Geometry check sheet. Reference: the model listing, model coordinates, mm. Give positions to 0.01 mm unless a question says otherwise; leave off trailing zeros. Write item = value, one per line. Start each with the question number.
1. Thickness scan on line 1 along X through (y, z) = (0.8, -6); line 2 along X through (y, z) = (0.6, -3); line 3 along Z through (x, y) = (-1.5, 1.25). Record the ranges inside material, lowest first.
2. Mould release check, pull along Z, two halves, no side actions. Record for faces 1 (the flat face through (4, 0, 13)), 2 (the conical face through (5.31, 2.94, -12.81)), 3 (the cylindrical face through (-13.22, 1.5, 1.74)): pulls with the +Z half, pulls with the -Z half, needs draft (parallel to the pull), parting line crosses it, or undercut.
3. Depth check by flat-ended pin: P1, Ø1.5, axis at y = 2, z = -11.5, coming from the +X side. Enter the tip coordinate at first touch or a pass-through.
```python
from build123d import *

# Parameters (mm, degrees)
SKETCH1_R       = 19.05
SKETCH1_R_2     = 13.335
EXTRUDE1_DEPTH  = 1.524
CHAMFER1_SIZE   = 1.27
CHAMFER1_SIZE2  = 1.065656532
SKETCH2_R       = 17.984343468
SKETCH2_R_2     = 13.335
EXTRUDE2_DEPTH  = 1.524
CHAMFER2_SIZE   = 4.426017378
CHAMFER2_SIZE_2 = 1.524
FILLET1_R       = 0.254


with BuildPart() as part:
    # Sketch1 → Extrude1 (new body)
    with BuildSketch(Plane(origin=(0, 0, 0), x_dir=(1, 0, 0), z_dir=(0, 1, 0))):
        with Locations(Location((0, 0, 0), (0, 0, 90))):
            Circle(SKETCH1_R)
        with Locations(Location((0, 0, 0), (0, 0, 90))):
            Circle(SKETCH1_R_2, mode=Mode.SUBTRACT)
    extrude(amount=EXTRUDE1_DEPTH)

    # Chamfer1
    chamfer1_edges = [part.edges().sort_by_distance(p)[0] for p in [
        (0, 1.524, 19.05),
    ]]
    chamfer1_side = [part.faces().sort_by_distance(p)[0] for p in [
        (0, 0.762, 19.05),
    ]]
    chamfer(chamfer1_edges, length=CHAMFER1_SIZE, length2=CHAMFER1_SIZE2, reference=chamfer1_side[0])

    # Sketch2 → Extrude2 (add)
    with BuildSketch(Plane(origin=(0, 1.524, 0), x_dir=(-1, 0, 0), z_dir=(0, 1, 0))):
        with Locations(Location((0, 0, 0), (0, 0, 270))):
            Circle(SKETCH2_R)
        with Locations(Location((0, 0, 0), (0, 0, 270))):
            Circle(SKETCH2_R_2, mode=Mode.SUBTRACT)
    extrude(amount=EXTRUDE2_DEPTH)

    # Chamfer2
    # the kernel refuses this chamfer: 4.426017378, 1.524 mm, written as the material it takes off along each edge
    with BuildSketch(Plane(origin=(0, 3.048, 0), x_dir=(0, 0, -1), z_dir=(1, 0, 0))) as chamfer2_piece_1:
        Polygon((17.984343468 - CHAMFER2_SIZE, 0), (17.984343468, -CHAMFER2_SIZE_2), (17.984343468, 0), align=None)
    revolve(axis=Axis((0, 3.048, 0), (0, 1, 0)), mode=Mode.SUBTRACT)

    # Fillet1
    fillet1_edges = [part.edges().sort_by_distance(p)[0] for p in [
        (0, 3.048, 13.55832609),
        (0, 1.524, 17.984343468),
        (0, 0.254, 19.05),
    ]]
    fillet(fillet1_edges, radius=FILLET1_R)


solid = part.part
```
Answers:
q1.line_1 = -17.6 to -11.91, 11.91 to 17.6
q1.line_2 = -18.52 to -12.99, 12.99 to 18.52
q1.line_3 = -18.15 to -13.25, 13.25 to 18.15
q2.face_1 = needs draft
q2.face_2 = parting line crosses it
q2.face_3 = undercut
q3.P1 = 14.32
